Input: part model. Units: mm. Frame: model coordinates. Face numbers are marked on the shaded views. A direction names the side the tool comes from. Coordinates: 2 decimals unless noted, no trailing zeros. Loops run counter-clockwise (first coordinate to the right, second up) from the corner with the lowest first, then second, coordinate; pieces in that order, holes last. Notation, with made-up numbers: (22.25, 46.25) - (27.25, 46.25) arc R24 cw to (27.25, 85.25) - close; hole circle Ø8 at (-18, 83). An arc over 180 degrees is marked (long way). Use a Markdown table: item, result. Add a question column.
1. Section query D-D on y = -3. Return the cut outline in (x, z), then the cut area to 3 significant figures.
2. Contact query for flat-ended pins moving along their axis: P1, Ø2, axis at y = 6, z = 3.5, coming from the +X side; P2, Ø1.5, axis at y = 4.5, z = 1.5, coming from the -X side; P3, Ø0.9, axis at x = 0, z = 1.5, coming from the +Y side; P4, Ø2.5, axis at x = 2.88, y = -5.53, coming from the -Z side. Output: stop coordinate, or through.
3. Draft query along X for the marked faces 1, 2 and 3. Return one class per face: released by +X, released by -X, zero draft, split by the parting line, or undercut.
4. Ray query, L1, parallel to X at y = 8, z = 2.25; L2, parallel to Y at x = 0, z = 4.5; L3, parallel to Y at x = 2.5, z = 4.5. Return the intervals inside material, ascending. Write a range as [from, to].
5. Section query C-C on z = 1.25. Return the cut outline in (x, y), then the cut area to 3 significant figures.
6. Section query B-B on y = 4. Return the cut outline in (x, z), then the cut area to 3 significant figures.
7. Section query A-A on z = 3.5. Return the cut outline in (x, y), then the cut area to 3 significant figures.
8. Access query for the marked faces 4, 5, 6, 7 and 8. Directions: +Z, -Z, +X, -X, +Y, -Y. A direction counts if a zero-diameter tool reaches every point of the face in a straight line with its end or side. Return the directions, or none.
Autodesk Inventor part; units mm, degrees
ref_plane "YZ Plane" through (0, 0, 0) normal (1, 0, 0) x (0, 1, 0)
ref_plane "XZ Plane" through (0, 0, 0) normal (0, 1, 0) x (-1, 0, 0)
ref_plane "XY Plane" through (0, 0, 0) normal (0, 0, 1) x (1, 0, 0)
sketch "Sketch1" plane through (0, 0, 0) normal (0, 0, 1) x (1, 0, 0)
  circle A0 centre (2.8817, -5.5305) radius 1
  circle A1 centre (-2.8817, -5.5305) radius 1
  line L0 (4.5, 12.6443) -> (5.9902, 11.1443)
  line L1 (3, 12.6443) -> (4.5, 12.6443)
  line L2 (3, -2.3557) -> (3, 12.6443)
  line L3 (-3, -2.3557) -> (3, -2.3557)
  line L4 (-3, 12.6443) -> (-3, -2.3557)
  line L5 (-4.5, 12.6443) -> (-3, 12.6443)
  line L6 (-5.9902, 11.1443) -> (-4.5, 12.6443)
  line L7 (-5.8406, -11.8556) -> (-5.9902, 11.1443)
  line L8 (-3.8536, -9.8557) -> (-5.8406, -11.8556)
  line L9 (-3.8536, -9.8557) -> (3.8536, -9.8557)
  line L10 (5.8406, -11.8556) -> (3.8536, -9.8557)
  line L11 (5.9902, 11.1443) -> (5.8406, -11.8556)
  line L12 (3.8536, -9.8557) -> (5.8536, -9.8557)
  line L13 (-3.8536, -9.8557) -> (-5.8535, -9.8687)
  point P0 (0, 0)
extrude "Extrusion1" add sketch "Sketch1" along normal blind 3 contours L0 L11 L12 L9 L13 L7 L6 L5 L4 L3 L2 L1
sketch "Sketch2" plane through (0, 0, 3) normal (0, 0, 1) x (1, 0, 0)
  line L0 (-3, -2.3557) -> (-3, 12.6443)
  line L1 (-3, 12.6443) -> (-4.5, 12.6443)
  line L2 (-4.5, 12.6443) -> (-5.9902, 11.1443)
  line L3 (-5.9902, 11.1443) -> (-5.8535, -9.8687)
  line L4 (-5.8535, -9.8687) -> (-3.8536, -9.8557)
  line L5 (-3.8536, -9.8557) -> (5.8536, -9.8557)
  line L6 (5.8536, -9.8557) -> (5.9902, 11.1443)
  line L7 (5.9902, 11.1443) -> (4.5, 12.6443)
  line L8 (4.5, 12.6443) -> (3, 12.6443)
  line L9 (3, 12.6443) -> (3, -2.3557)
  line L10 (3, -2.3557) -> (-3, -2.3557)
  circle A0 centre (-2.8817, -5.5305) radius 1
  circle A1 centre (2.8817, -5.5305) radius 1
  line L11 (3, 12.6443) -> (3, -2.3557)
  line L12 (-3, 12.6443) -> (3, 12.6443)
  point P0 (0, 0)
extrude "Extrusion2" add sketch "Sketch2" along normal blind 3
sketch "Sketch3" plane through (0, 0, 6) normal (0, 0, 1) x (1, 0, 0)
  line L0 (-5.8535, -9.8687) -> (-3.8536, -9.8557)
  line L1 (-3.8536, -9.8557) -> (5.8536, -9.8557)
  line L2 (5.8536, -9.8557) -> (5.9902, 11.1443)
  line L3 (5.9902, 11.1443) -> (4.5, 12.6443)
  line L4 (4.5, 12.6443) -> (-4.5, 12.6443)
  line L5 (-4.5, 12.6443) -> (-5.9902, 11.1443)
  line L6 (-5.9902, 11.1443) -> (-5.8535, -9.8687)
  circle A0 centre (2.8817, -5.5305) radius 1
  circle A1 centre (-2.8817, -5.5305) radius 1
  line L7 (-5.8535, -9.8687) -> (-3.8536, -9.8557)
  arc A2 (5.8536, -9.8557) -> (-5.8535, -9.8687) centre (0.0154, -23.6729) ccw
  point P0 (0, 0)
  dimension "d4" = 15
extrude "Extrusion3" cut sketch "Sketch3" against normal blind 8 contours A2 L1 L0
chamfer "Chamfer1" distance 3 angle 45 2 edges at (5.8536, -9.8557, 3) (-5.8535, -9.8687, 3)
fillet "Fillet1" radius 2 2 edges at (5.2451, 11.8943, 6) (-5.2451, 11.8943, 6)
fillet "Fillet2" radius 1 3 edges at (-4.4311, -7.9228, 6) (-0.0013, -8.6729, 6) (4.4302, -7.913, 6)
sketch "Sketch4" plane through (0, 0, 6) normal (0, 0, 1) x (1, 0, 0)
  line L0 (-1, 8.1443) -> (-1, 2.1443)
  arc A0 (-1, 2.1443) -> (1, 2.1443) centre (0, 2.1443) ccw
  line L1 (1, 2.1443) -> (1, 8.1443)
  arc A1 (1, 8.1443) -> (-1, 8.1443) centre (0, 8.1443) ccw
  line L2 (5.9719, 8.3251) -> (1.6807, 12.6443)
  line L3 (5.9719, 8.3251) -> (5.8537, -9.8477)
  line L4 (3.4979, -11.4182) -> (5.8537, -9.8477)
  spline S0 degree 3 poles (3.7471, -14.0453) (3.5143, -13.7817) (3.313, -13.4738) (3.0785, -12.9028) (3.0205, -12.6553) (3.011, -12.2509) (3.0346, -12.0815) (3.1344, -11.8203) (3.188, -11.725) (3.325, -11.5531) (3.4063, -11.4793) (3.4979, -11.4182) knots 0 0 0 0 0.105501 0.105501 0.185956 0.185956 0.244407 0.244407 0.282215 0.282215 0.320119 0.320119 0.320119 0.320119
  arc A2 (-3.7471, -14.0453) -> (3.7471, -14.0453) centre (0, -17.3557) ccw
  spline S1 degree 3 poles (-3.4979, -11.4182) (-3.3811, -11.4961) (-3.2816, -11.5944) (-3.1273, -11.8263) (-3.0754, -11.9539) (-3.0096, -12.2519) (-3.0068, -12.4209) (-3.0565, -12.825) (-3.1338, -13.0604) (-3.3668, -13.5541) (-3.5446, -13.816) (-3.7471, -14.0453) knots 0 0 0 0 0.042129 0.042129 0.083567 0.083567 0.133564 0.133564 0.205298 0.205298 0.296261 0.296261 0.296261 0.296261
  line L5 (-5.8537, -9.8477) -> (-3.4979, -11.4182)
  line L6 (-5.8537, -9.8477) -> (-5.9719, 8.3251)
  line L7 (-1.6807, 12.6443) -> (-5.9719, 8.3251)
  line L8 (-1.6807, 12.6443) -> (1.6807, 12.6443)
  circle A3 centre (0, -17.3557) radius 1.5
  circle A4 centre (-2.8817, -5.5305) radius 1
  circle A5 centre (2.8817, -5.5305) radius 1
  point P0 (0, 0)
extrude "Extrusion4" cut sketch "Sketch4" against normal blind 8 contours A1 L1 A0 L0
chamfer "Chamfer2" distance 1 angle 45 4 edges at (-1, 5.1443, 6) (0, 9.1443, 6) (1, 5.1443, 6) (0, 1.1443, 6)
properties part number "arm_linkage_3"
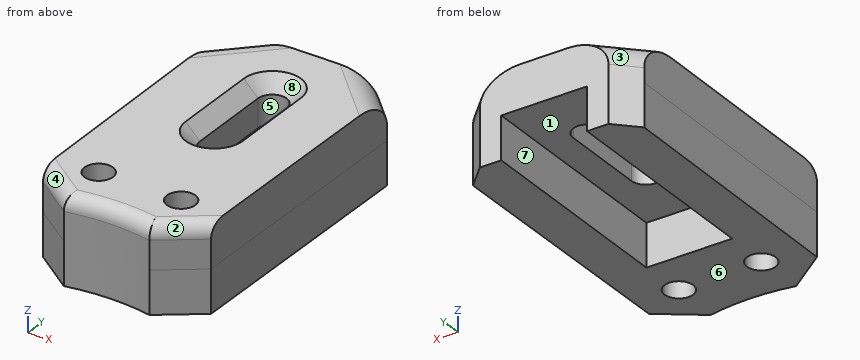
Resolved:
| question | item | result |
|---|---|---|
| 1 | outline | (-5.9, 0) - (5.9, 0) - (5.9, 6) - (-5.9, 6) - close |
| 1 | area | 70.8 mm² |
| 2 | P1 | x = 5.96 |
| 2 | P2 | x = -5.95 |
| 2 | P3 | y = -2.36 |
| 2 | P4 | z = 0 |
| 3 | face 1 | undercut |
| 3 | face 2 | released by +X |
| 3 | face 3 | released by -X |
| 4 | L1 | [-5.97, -3], [3, 5.97] |
| 4 | L2 | [-8.67, 1.14], [9.14, 12.64] |
| 4 | L3 | [-8.88, -6.45], [-4.61, 12.64] |
| 5 | outline | (-5.99, 11.14) - (-5.87, -6.87) - (-2.99, -8.98) arc R15 cw to (2.99, -8.97) - (5.87, -6.86) - (5.99, 11.14) - (4.5, 12.64) - (3, 12.64) - (3, -2.36) - (-3, -2.36) - (-3, 12.64) - (-4.5, 12.64) - close; hole circle Ø2 at (-2.88, -5.53); hole circle Ø2 at (2.88, -5.53) |
| 5 | area | 151 mm² |
| 6 | outline | (-5.94, 0) - (-3, 0) - (-3, 3) - (-1, 3) - (-1, 5) - (-2, 6) - (-5.94, 6) - close; (1, 3) - (3, 3) - (3, 0) - (5.94, 0) - (5.94, 6) - (2, 6) - (1, 5) - close |
| 6 | area | 46.3 mm² |
| 7 | outline | (-5.99, 11.14) - (-5.87, -6.87) - (-2.99, -8.98) arc R15 cw to (2.99, -8.97) - (5.87, -6.86) - (5.99, 11.14) - (4.5, 12.64) - (-4.5, 12.64) - close; hole circle Ø2 at (-2.88, -5.53); hole (-1, 2.14) arc R1 ccw to (1, 2.14) - (1, 8.14) arc R1 ccw to (-1, 8.14) - close; hole circle Ø2 at (2.88, -5.53) |
| 7 | area | 225 mm² |
| 8 | face 4 | +Z, -X, -Y |
| 8 | face 5 | +Z, -Z |
| 8 | face 6 | -Z, +X, -X, +Y, -Y |
| 8 | face 7 | -Z, +Y |
| 8 | face 8 | +Z |
